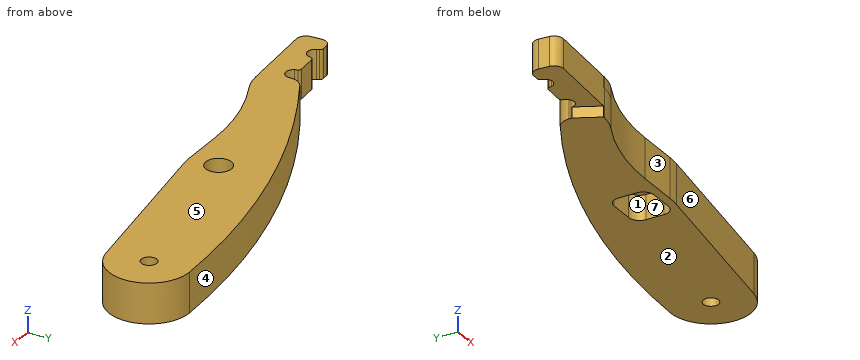
```python
from build123d import *

# Parameters (mm, degrees)
BOSS_EXTRUDE1_DEPTH          = 3.5
BOSS_EXTRUDE2_DEPTH          = 9.5
BOSS_EXTRUDE2_DEPTH_BACK     = 3.5
CUT_EXTRUDE1_DEPTH           = 268.941422383
SKETCH4_W                    = 15
SKETCH4_H                    = 13
CUT_EXTRUDE2_DEPTH           = 8
F_5_16_CLEARANCE_HOLE1_D     = 8.4
F_5_16_CLEARANCE_HOLE1_DEPTH = 13
FILLET1_R                    = 1
FILLET2_R                    = 3
FILLET3_R                    = 3.5
FILLET4_R                    = 5
FILLET5_R                    = 18
FILLET6_R                    = 27.432772437
SKETCH9_R                    = 2.51
CUT_EXTRUDE3_DEPTH           = 268.881580074
CUT_EXTRUDE4_DEPTH           = 3.5


with BuildPart() as part:
    # Sketch1 → Boss-Extrude1 (new body)
    with BuildSketch(Plane.XY.offset(47.8)):
        with BuildLine():
            Line((-55.017772963, 219.948002855), (-50.996862784, 212.056522295))
            Line((-50.996862784, 212.056522295), (-46.846659232, 212.346732798))
            ThreePointArc((-46.846659232, 212.346732798), (-30.700707895, 218.653781383), (-13.5, 220.8))
            Line((-13.5, 220.8), (2.038607139, 220.8))
            Line((2.038607139, 220.8), (60.876238897, 229.593342983))
            ThreePointArc((60.876238897, 229.593342983), (71.950599997, 243.603343771), (58.674027502, 255.547137919))
            ThreePointArc((58.674027502, 255.547137919), (-0.148756736, 246.886614708), (-54.989372002, 223.916383428))
            Line((-54.989372002, 223.916383428), (-54.989372002, 220.323766337))
            ThreePointArc((-54.989372002, 220.323766337), (-54.996482354, 220.13534871), (-55.017772963, 219.948002855))
        make_face()
    extrude(amount=-BOSS_EXTRUDE1_DEPTH)

    # Sketch2 → Boss-Extrude2 (add, two sides: drawn at the far end of the back side and taken through both)
    with BuildSketch(Plane(origin=(0, 0, 44.3), x_dir=(-1, 0, 0), z_dir=(0, 0, -1)).offset(-BOSS_EXTRUDE2_DEPTH_BACK)):
        with BuildLine():
            Line((60.44632379, 220.818705454), (79.484610639, 219.487418749))
            Line((79.484610639, 219.487418749), (78.828899786, 210.110316677))
            Line((78.828899786, 210.110316677), (46.846659232, 212.346732798))
            ThreePointArc((46.846659232, 212.346732798), (30.700707895, 218.653781383), (13.5, 220.8))
            Line((13.5, 220.8), (-2.038607139, 220.8))
            Line((-2.038607139, 220.8), (-60.876238897, 229.593342983))
            ThreePointArc((-60.876238897, 229.593342983), (-71.950599997, 243.603343771), (-58.674027502, 255.547137919))
            ThreePointArc((-58.674027502, 255.547137919), (0.148756736, 246.886614708), (54.989372002, 223.916383428))
            Line((54.989372002, 223.916383428), (54.989372002, 220.323766337))
            ThreePointArc((54.989372002, 220.323766337), (56.969592775, 217.878397335), (59.773235646, 219.306924729))
            Line((59.773235646, 219.306924729), (60.44632379, 220.818705454))
        make_face()
    extrude(amount=BOSS_EXTRUDE2_DEPTH + BOSS_EXTRUDE2_DEPTH_BACK)

    # Sketch3 → Cut-Extrude1 (cut, through all)
    with BuildSketch(Plane(origin=(0, 0, 34.8), x_dir=(-1, 0, 0), z_dir=(0, 0, -1))):
        with BuildLine():
            Line((73.913438469, 219.876993058), (68.097193955, 220.283704494))
            Line((68.097193955, 220.283704494), (68.55333244, 218.692960552))
            ThreePointArc((68.55333244, 218.692960552), (70.782095496, 216.888143816), (73.240350324, 218.365212333))
            Line((73.240350324, 218.365212333), (73.913438469, 219.876993058))
        make_face()
    extrude(amount=-CUT_EXTRUDE1_DEPTH, mode=Mode.SUBTRACT)

    # Sketch4 → Cut-Extrude2 (cut)
    with BuildSketch(Plane(origin=(0, 0, 34.8), x_dir=(-1, 0, 0), z_dir=(0, 0, -1))):
        with Locations((0, 230.1)):
            Rectangle(SKETCH4_W, SKETCH4_H)
    extrude(amount=-CUT_EXTRUDE2_DEPTH, mode=Mode.SUBTRACT)

    # 5/16 Clearance Hole1
    with Locations(Plane.XY.offset(47.8)):
        with Locations((0, 230.1)):
            Hole(F_5_16_CLEARANCE_HOLE1_D / 2, depth=F_5_16_CLEARANCE_HOLE1_DEPTH)

    # Fillet1
    fillet1_edges = [part.edges().sort_by_distance(p)[0] for p in [
        (-60.44632379, 220.818705454, 41.3),
        (-73.913438469, 219.876993058, 41.3),
        (-68.097193955, 220.283704494, 41.3),
    ]]
    fillet(fillet1_edges, radius=FILLET1_R)

    # Fillet2
    fillet2_edges = [part.edges().sort_by_distance(p)[0] for p in [
        (-79.484610639, 219.487418749, 41.3),
        (-78.828899786, 210.110316677, 41.3),
    ]]
    fillet(fillet2_edges, radius=FILLET2_R)

    # Fillet3
    fillet3_edges = [part.edges().sort_by_distance(p)[0] for p in [
        (-7.5, 236.6, 38.8),
        (-7.5, 223.6, 38.8),
        (7.5, 223.6, 38.8),
        (7.5, 236.6, 38.8),
    ]]
    fillet(fillet3_edges, radius=FILLET3_R)

    # Fillet4
    fillet4_edges = [part.edges().sort_by_distance(p)[0] for p in [
        (-54.989372002, 223.916383428, 41.3),
    ]]
    fillet(fillet4_edges, radius=FILLET4_R)

    # Fillet5
    fillet5_edges = [part.edges().sort_by_distance(p)[0] for p in [
        (-46.846659232, 212.346732798, 41.3),
    ]]
    fillet(fillet5_edges, radius=FILLET5_R)

    # Fillet6
    fillet6_edges = [part.edges().sort_by_distance(p)[0] for p in [
        (2.038607139, 220.8, 41.3),
    ]]
    fillet(fillet6_edges, radius=FILLET6_R)

    # Sketch9 → Cut-Extrude3 (cut, through all)
    with BuildSketch(Plane(origin=(0, 0, 34.8), x_dir=(-1, 0, 0), z_dir=(0, 0, -1))):
        with Locations((-58.947326081, 242.5)):
            Circle(SKETCH9_R)
    extrude(amount=-CUT_EXTRUDE3_DEPTH, mode=Mode.SUBTRACT)

    # Sketch10 → Cut-Extrude4 (cut)
    with BuildSketch(Plane(origin=(0, 0, 34.8), x_dir=(-1, 0, 0), z_dir=(0, 0, -1))):
        Polygon((50.996862784, 212.056522295), (55.017772963, 219.948002855), (56.636135003, 223.124217196), (80.862126047, 221.430170876), (79.948532306, 208.3651717), (50.433855775, 210.429038936), align=None)
    extrude(amount=-CUT_EXTRUDE4_DEPTH, mode=Mode.SUBTRACT)


solid = part.part
```
Model file for the job. Use its own axes, mm. Face numbers are marked on the shaded views. A direction names the side the tool comes from. Coordinates: 2 decimals unless noted, no trailing zeros. Loops run counter-clockwise (first coordinate to the right, second up) from the corner with the lowest first, then second, coordinate; pieces in that order, holes last. Notation, with made-up numbers: (68.25, 2) - (119.25, 2) arc R17 cw to (119.25, 15) - close; hole circle Ø4 at (-13, 64.5). An arc over 180 degrees is marked (long way). Answer as a JSON object with one key per item and string values. Group by question number.
(1) Probe line 1 along Y through (x, z) = (-2, 47.25); line 2 along X through (y, z) = (233, 40.75); line 3 along Y through (x, z) = (61, 39). List the from-to ranges inside material, lowest first.
(2) Flat gauge pins, fed straight in: pin 1 (3 mm diameter, centred on x = -58.5, y = 216, fed in from -Z); pin 2 (6 mm diameter, centred on x = 58.95, y = 242.5, fed in from -Z); pin 3 (3 mm diameter, centred on y = 231, z = 39, fed in from +X); pin 4 (5 mm diameter, centred on x = 1.5, z = 38, fed in from -Y). Where does each tip first touch, or does it go through?
(3) Cut at A-A (z = 41.5). State how many separate pieces and enclosed holes the cut face has, then the cut area to 3 significant figures.
(4) Cut at C-C (x = 38.5). Give the cut face in (y, z).
(5) Tool access for the marked faces 1, 2 and 3: list every direction of +Z, -Z, +X, -X, +Y, -Y with a clear straight run to the whole face (end or side of a thin tool).
(6) Cut at B-B (y = 242.5). Give the cut face in (x, z).
(7) Two-plate mould, pull along Y, no slides. Class the marked faces 4, 5, 6 and 7: released by +Y, released by -Y, zero draft, split by the parting line, or undercut.
Geometry says:
{
 "1": {"line 1": "y = 220.8 to 226.41, 233.79 to 246.36", "line 2": "x = -37.57 to -7.5, 7.5 to 67.89", "line 3": "y = 229.61 to 241.06, 243.94 to 255.39"},
 "2": {"pin 1": "stops at z = 38.3", "pin 2": "stops at z = 34.8", "pin 3": "stops at x = 67.33", "pin 4": "stops at y = 220.8"},
 "3": {"separate pieces": "1", "enclosed holes": "2", "area": "2,930 mm^2"},
 "4": {"outline": "(226.25, 34.8) - (254.27, 34.8) - (254.27, 47.8) - (226.25, 47.8) - close"},
 "5": {"face 1": "-Z", "face 2": "-Z, +X, -X, +Y, -Y", "face 3": "+Z, -Z, +X, -Y"},
 "6": {"outline": "(-14.21, 34.8) - (56.44, 34.8) - (56.44, 47.8) - (-14.21, 47.8) - close; (61.46, 34.8) - (72, 34.8) - (72, 47.8) - (61.46, 47.8) - close"},
 "7": {"face 4": "released by +Y", "face 5": "zero draft", "face 6": "released by -Y", "face 7": "undercut"}
}
